Could you check a few things on this model? Use its own coordinates, in mm. Face numbers are marked on the shaded views. Give positions to 0.01 mm unless a question says otherwise; leave off trailing zeros. Write each loop counter-clockwise with the first axis right and the second up, starting at its lowest first coordinate (ties: lowest second). Pieces come first, ordered by that corner, then holes. Notation, with made-up numbers: (74, 39.5) - (107, 39.5) arc R26 cw to (107, 57.5) - close; hole circle Ø9 at (-30.5, -18). An arc over 180 degrees is marked (long way). Use one line per item in the form item = value.
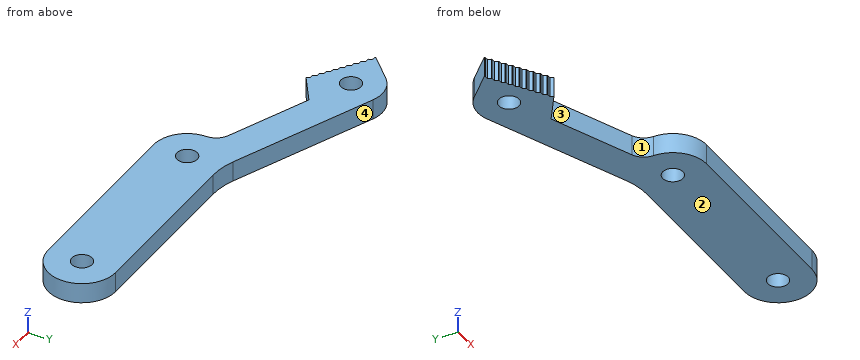
```python
from build123d import *

# Parameters (mm, degrees)
SKETCH1_R            = 1.5
BOSS_EXTRUDE1_DEPTH  = 3
CUT_EXTRUDE1_DEPTH   = 23
LPATTERN1_COUNT      = 2
LPATTERN1_PITCH      = 10
LPATTERN1_COUNT_DIR2 = 10
LPATTERN1_PITCH_DIR2 = 1


with BuildPart() as part:
    # Sketch1 → Boss-Extrude1 (new body)
    with BuildSketch(Plane.XY):
        with BuildLine():
            Line((-11.510876326, 5), (13.5, 5))
            ThreePointArc((13.5, 5), (18.5, 0), (13.5, -5))
            Line((13.5, -5), (-13.5, -5))
            ThreePointArc((-13.5, -5), (-17.032859244, -3.538206546), (-18.499994281, -0.007562225))
            ThreePointArc((-18.499994281, -0.007562225), (-18.922368323, 1.379153788), (-20.043282841, 2.298355494))
            Line((-20.043282841, 2.298355494), (-32.109838269, 7.296486403))
            Line((-32.109838269, 7.296486403), (-36.245393033, 4.48629303))
            Line((-36.245393033, 4.48629303), (-44.606456533, 9.97196684))
            Line((-44.606456533, 9.97196684), (-41.286860538, 13.369433901))
            ThreePointArc((-41.286860538, 13.369433901), (-38.910252818, 14.666448531), (-36.215040659, 14.408877911))
            Line((-36.215040659, 14.408877911), (-15.33771065, 5.761204675))
            ThreePointArc((-15.33771065, 5.761204675), (-13.461779546, 5.192147196), (-11.510876326, 5))
        make_face()
        with Locations((-13.5, 0)):
            Circle(SKETCH1_R, mode=Mode.SUBTRACT)
        with Locations((13.5, 0)):
            Circle(SKETCH1_R, mode=Mode.SUBTRACT)
        with Locations((-37.982807612, 10.141110958)):
            Circle(SKETCH1_R, mode=Mode.SUBTRACT)
    extrude(amount=BOSS_EXTRUDE1_DEPTH)

    # Sketch3 → Cut-Extrude1 (cut)
    with BuildSketch(Plane.XY.offset(3)):
        Polygon((-36.470295857, 4.932856261), (-36.969482372, 4.961366317), (-36.245393033, 4.48629303), align=None)
    cut_extrude1 = extrude(amount=-CUT_EXTRUDE1_DEPTH, mode=Mode.SUBTRACT)

    # LPattern1: Cut-Extrude1 2 × 10
    with Locations(*[Vector(-0.8361063499961565, 0.5485673809990023, 0) * (i * LPATTERN1_PITCH) + Vector(0.8361063499961561, -0.548567380999003, 0) * (j * LPATTERN1_PITCH_DIR2) for i in range(LPATTERN1_COUNT) for j in range(LPATTERN1_COUNT_DIR2) if (i, j) != (0, 0)]):
        add(cut_extrude1, mode=Mode.SUBTRACT)


solid = part.part
```
1. Imagine slicing it at C-C, the plane x = 8. List the corners of the cut face in (y, z) for me.
Response values:
outline = (-5, 0) - (5, 0) - (5, 3) - (-5, 3) - close
2. Imagine slicing it at A-A, the plane y = -3. List the corners of the cut face in (x, z) for me.
Response values:
outline = (-17.5, 0) - (17.5, 0) - (17.5, 3) - (-17.5, 3) - close
3. If we mould it in two halves opening along X, with no side actions, what happens to the marked faces 1, 2, 3 and 4? For each: pulls with the +X half, pulls with the -X half, needs draft (parallel to the pull), parting line crosses it, or undercut.
Response values:
face_1 = pulls with the -X half
face_2 = needs draft
face_3 = undercut
face_4 = pulls with the +X half
4. If I drill on line 1 (Y direction, x = 13.5, z = 1.6); line 2 (Y direction, x = 9.5, z = 2); line 3 (X direction, y = 9.75, z = 1.95), over which ranges is the centre line in solid material (lowest first)? Write a range as from..to.
Response values:
line_1 = -5..-1.5, 1.5..5
line_2 = -5..5
line_3 = -43.93..-39.43, -36.53..-24.97
5. Imagine slicing it at B-B, the plane z = 0.95. State how many separate pieces and enclosed holes the cut face has, and give its area (3 significant figures).
Response values:
separate_pieces = 1
enclosed_holes = 3
area = 494 mm²
6. For pin 1 (5 mm diameter, centred on x = -37.5, y = 11.5, fed in from -Z); pin 2 (1 mm diameter, centred on y = 12.5, z = 2, fed in from +X), each with a flat end and sliding along its axis, tell me the tip position at first contact or that it passes through.
Response values:
pin_1 = 0
pin_2 = -30.4
